The model under review builds one solid part; all positions refer to its coordinate system, in mm. Face numbers are marked on the shaded views. Give positions to 0.01 mm unless a question says otherwise; leave off trailing zeros. Order: outer loops, then holes, each group sorted by start corner. A loop starts at its lowest first (then second) coordinate and runs counter-clockwise, first axis right, second up. Notation, with made-up numbers: (-22, 24) - (32, 24) arc R25 ccw to (32, 46) - close; hole circle Ø4 at (6, 44). An arc over 180 degrees is marked (long way). Use CSV: the item, a comma, the result in double quotes.
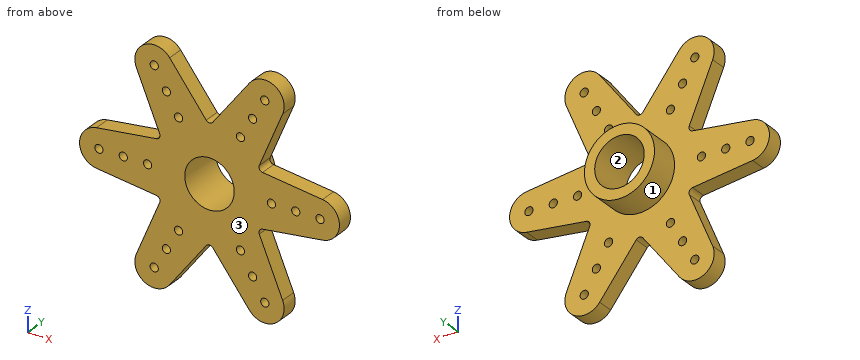
```python
from build123d import *

# Parameters (mm, degrees)
SKETCH1_R           = 3
SKETCH1_R_2         = 0.5
BOSS_EXTRUDE1_DEPTH = 2
SKETCH2_R           = 4.25
SKETCH2_R_2         = 3
BOSS_EXTRUDE2_DEPTH = 3.65


with BuildPart() as part:
    # Sketch1 → Boss-Extrude1 (new body)
    with BuildSketch(Plane(origin=(0, 0, 0), x_dir=(1, 0, 0), z_dir=(0, 1, 0))):
        with BuildLine():
            Line((13.696134198, 2.331266724), (6.432183252, 3.253985803))
            ThreePointArc((6.432183252, 3.253985803), (6.062177826, 3.5), (6.034125995, 3.943441197))
            Line((6.034125995, 3.943441197), (8.867003305, 10.695566787))
            ThreePointArc((8.867003305, 10.695566787), (7.875, 13.63990011), (4.829130893, 13.026833511))
            Line((4.829130893, 13.026833511), (0.398057257, 7.197427))
            ThreePointArc((0.398057257, 7.197427), (0, 7), (-0.398057257, 7.197427))
            Line((-0.398057257, 7.197427), (-4.829130893, 13.026833511))
            ThreePointArc((-4.829130893, 13.026833511), (-7.875, 13.63990011), (-8.867003305, 10.695566787))
            Line((-8.867003305, 10.695566787), (-6.034125995, 3.943441197))
            ThreePointArc((-6.034125995, 3.943441197), (-6.062177826, 3.5), (-6.432183252, 3.253985803))
            Line((-6.432183252, 3.253985803), (-13.696134198, 2.331266724))
            ThreePointArc((-13.696134198, 2.331266724), (-15.75, 0), (-13.696134198, -2.331266724))
            Line((-13.696134198, -2.331266724), (-6.432183252, -3.253985803))
            ThreePointArc((-6.432183252, -3.253985803), (-6.062177826, -3.5), (-6.034125995, -3.943441197))
            Line((-6.034125995, -3.943441197), (-8.867003305, -10.695566787))
            ThreePointArc((-8.867003305, -10.695566787), (-7.875, -13.63990011), (-4.829130893, -13.026833511))
            Line((-4.829130893, -13.026833511), (-0.398057257, -7.197427))
            ThreePointArc((-0.398057257, -7.197427), (0, -7), (0.398057257, -7.197427))
            Line((0.398057257, -7.197427), (4.829130893, -13.026833511))
            ThreePointArc((4.829130893, -13.026833511), (7.875, -13.63990011), (8.867003305, -10.695566787))
            Line((8.867003305, -10.695566787), (6.034125995, -3.943441197))
            ThreePointArc((6.034125995, -3.943441197), (6.062177826, -3.5), (6.432183252, -3.253985803))
            Line((6.432183252, -3.253985803), (13.696134198, -2.331266724))
            ThreePointArc((13.696134198, -2.331266724), (15.75, 0), (13.696134198, 2.331266724))
        make_face()
        with Locations(Location((0, 0, 0), (0, 0, 270))):
            Circle(SKETCH1_R, mode=Mode.SUBTRACT)
        with Locations(Location((7.5, 0, 0), (0, 0, 270))):
            Circle(SKETCH1_R_2, mode=Mode.SUBTRACT)
        with Locations(Location((10.45, 0, 0), (0, 0, 270))):
            Circle(SKETCH1_R_2, mode=Mode.SUBTRACT)
        with Locations(Location((13.4, 0, 0), (0, 0, 270))):
            Circle(SKETCH1_R_2, mode=Mode.SUBTRACT)
        with Locations(Location((3.75, -6.495190528, 0), (0, 0, 270))):
            Circle(SKETCH1_R_2, mode=Mode.SUBTRACT)
        with Locations(Location((5.225, -9.04996547, 0), (0, 0, 270))):
            Circle(SKETCH1_R_2, mode=Mode.SUBTRACT)
        with Locations(Location((6.7, -11.604740411, 0), (0, 0, 270))):
            Circle(SKETCH1_R_2, mode=Mode.SUBTRACT)
        with Locations(Location((-3.75, -6.495190528, 0), (0, 0, 270))):
            Circle(SKETCH1_R_2, mode=Mode.SUBTRACT)
        with Locations(Location((-5.225, -9.04996547, 0), (0, 0, 270))):
            Circle(SKETCH1_R_2, mode=Mode.SUBTRACT)
        with Locations(Location((-6.7, -11.604740411, 0), (0, 0, 270))):
            Circle(SKETCH1_R_2, mode=Mode.SUBTRACT)
        with Locations(Location((-7.5, 0, 0), (0, 0, 270))):
            Circle(SKETCH1_R_2, mode=Mode.SUBTRACT)
        with Locations(Location((-10.45, 0, 0), (0, 0, 270))):
            Circle(SKETCH1_R_2, mode=Mode.SUBTRACT)
        with Locations(Location((-13.4, 0, 0), (0, 0, 270))):
            Circle(SKETCH1_R_2, mode=Mode.SUBTRACT)
        with Locations(Location((-3.75, 6.495190528, 0), (0, 0, 270))):
            Circle(SKETCH1_R_2, mode=Mode.SUBTRACT)
        with Locations(Location((-5.225, 9.04996547, 0), (0, 0, 270))):
            Circle(SKETCH1_R_2, mode=Mode.SUBTRACT)
        with Locations(Location((-6.7, 11.604740411, 0), (0, 0, 270))):
            Circle(SKETCH1_R_2, mode=Mode.SUBTRACT)
        with Locations(Location((3.75, 6.495190528, 0), (0, 0, 270))):
            Circle(SKETCH1_R_2, mode=Mode.SUBTRACT)
        with Locations(Location((5.225, 9.04996547, 0), (0, 0, 270))):
            Circle(SKETCH1_R_2, mode=Mode.SUBTRACT)
        with Locations(Location((6.7, 11.604740411, 0), (0, 0, 270))):
            Circle(SKETCH1_R_2, mode=Mode.SUBTRACT)
    extrude(amount=BOSS_EXTRUDE1_DEPTH)

    # Sketch2 → Boss-Extrude2 (add)
    with BuildSketch(Plane(origin=(0, 2, 0), x_dir=(-1, 0, 0), z_dir=(0, 1, 0))):
        with Locations(Location((0, 0, 0), (0, 0, 90))):
            Circle(SKETCH2_R)
        with Locations(Location((0, 0, 0), (0, 0, 90))):
            Circle(SKETCH2_R_2, mode=Mode.SUBTRACT)
    extrude(amount=BOSS_EXTRUDE2_DEPTH)


solid = part.part
```
Item 1: Clearance check with flat-ended pins moving along their axes: pin 1 (1 mm diameter, centred on y = 1.5, z = 10, fed in from -X); pin 2 (2 mm diameter, centred on x = -2.5, y = 4, fed in from +Z); pin 3 (9.5 mm diameter, centred on x = 0, z = 0, fed in from -Y); pin 4 (1.5 mm diameter, centred on x = -3, z = -4.5, fed in from +Y). State where each tip first meets the part, or that it passes through.
Results list:
pin 1,"stops at x = -8.78"
pin 2,"stops at z = 3.98"
pin 3,"stops at y = 0"
pin 4,"stops at y = 2"
Item 2: Take a section at A-A, the plane x = -10.45. Give the boundary of the cut face in (y, z), and give its area (3 significant figures).
Results list:
outline,"(0, -2.74) - (2, -2.74) - (2, -0.5) - (0, -0.5) - close; (0, 0.5) - (2, 0.5) - (2, 2.74) - (0, 2.74) - close"
area,"8.97 mm2"
Item 3: Wall thickness on L1, parallel to X at y = 1.05, z = 9; L2, parallel to Y at x = -5, z = 11; L3, parallel to Z at x = -2, y = 2.5: over which ranges is each line inside the solid? List them lowest first.
Results list:
L1,"x = -8.16 to -5.72, -4.73 to -1.77, 1.77 to 4.73, 5.72 to 8.16"
L2,"y = 0 to 2"
L3,"z = -3.75 to -2.24, 2.24 to 3.75"
Item 4: Mouldability with a two-part tool opening along X and no side actions: class the marked faces 1, 2 and 3 as pulls with the +X half, pulls with the -X half, needs draft (parallel to the pull), parting line crosses it, or undercut.
Results list:
face 1,"parting line crosses it"
face 2,"undercut"
face 3,"needs draft"
Item 5: Take a section at D-D, the plane y = 4.15. Give the boundary of the cut face in (x, z).
Results list:
outline,"circle Ø8.5 at (0, 0); hole circle Ø6 at (0, 0)"
Item 6: Take a section at B-B, the plane z = -10.25. Give the boundary of the cut face in (x, y), and give its area (3 significant figures).
Results list:
outline,"(-8.68, 0) - (-2.72, 0) - (-2.72, 2) - (-8.68, 2) - close; (2.72, 0) - (8.68, 0) - (8.68, 2) - (2.72, 2) - close"
area,"23.8 mm2"
Item 7: Take a section at C-C, the plane x = -3.75. Give the boundary of the cut face in (y, z), and give its area (3 significant figures).
Results list:
outline,"(0, -11.61) - (2, -11.61) - (2, -7) - (0, -7) - close; (0, -6) - (2, -6) - (2, -2) - (5.65, -2) - (5.65, 2) - (2, 2) - (2, 6) - (0, 6) - close; (0, 7) - (2, 7) - (2, 11.61) - (0, 11.61) - close"
area,"57.0 mm2"
